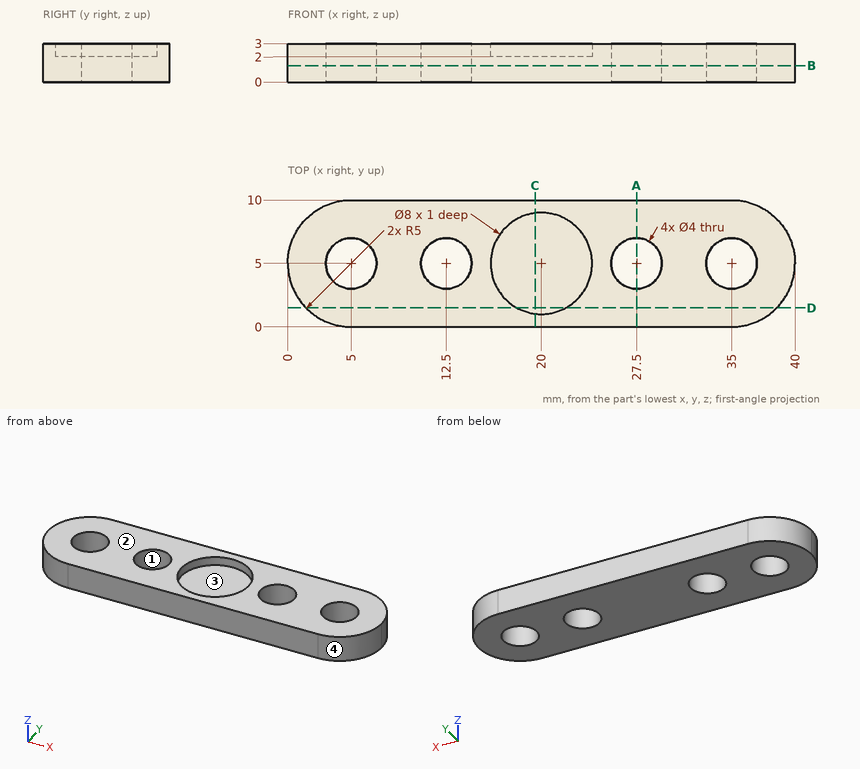
Source: three-view drawing plus pictorial views. Frame: mm from the lowest corner of the part. Round coordinates to 2 decimals unless told otherwise and drop trailing zeros. Write each loop counter-clockwise with the first axis right and the second up, starting at its lowest first coordinate (ties: lowest second). Pieces come first, ordered by that corner, then holes. Notation, with made-up numbers: M 68,72 L 105,72 A25 ccw 105,108 Z; hole C 14.5,60.5 d8. An arc over 180 degrees is marked long. Write item = value, one per line.
Item 1: Section query C-C on x = 19.5. Return loops of the section in (y, z).
Findings:
outline = M 0,0 L 10,0 L 10,3 L 8.97,3 L 8.97,2 L 1.03,2 L 1.03,3 L 0,3 Z
Item 2: Section query B-B on z = 1.3. State how many separate pieces and enclosed holes the cut face has, then the cut area to 3 significant figures.
Findings:
separate_pieces = 1
enclosed_holes = 4
area = 328 mm^2
Item 3: Pull-direction query (X, two-part tool) for the marked faces 1, 2, 3 and 4; classes: pulls with the +X half, pulls with the -X half, needs draft (parallel to the pull), parting line crosses it, or undercut.
Findings:
face_1 = undercut
face_2 = needs draft
face_3 = undercut
face_4 = pulls with the +X half
Item 4: Section query A-A on x = 27.5. Return loops of the section in (y, z).
Findings:
outline = M 0,0 L 3,0 L 3,3 L 0,3 Z; M 7,0 L 10,0 L 10,3 L 7,3 Z
Item 5: Pin query (flat end, axial travel): P1, Ø5, axis at x = 20, y = 5, coming from the +Z side. Return the tip coordinate at first contact, or that it passes through.
Findings:
P1 = 2
Item 6: Section query D-D on y = 1.5. Return loops of the section in (x, z), then the cut area to 3 significant figures.
Findings:
outline = M 1.43,0 L 38.57,0 L 38.57,3 L 21.94,3 L 21.94,2 L 18.06,2 L 18.06,3 L 1.43,3 Z
area = 108 mm^2
Item 7: Material intervals for line 1 along Y through (x, z) = (35, 1.5); line 2 along X through (y, z) = (4.75, 2.3); line 3 along X through (y, z) = (6.75, 1.55), sorted ascending. Write a range as [from, to].
Findings:
line_1 = [0, 3], [7, 10]
line_2 = [0.01, 3.02], [6.98, 10.52], [14.48, 16.01], [23.99, 25.52], [29.48, 33.02], [36.98, 39.99]
line_3 = [0.32, 4.03], [5.97, 11.53], [13.47, 26.53], [28.47, 34.03], [35.97, 39.68]
